Geometry: final body of the model. Coordinates: model frame, mm. A direction names the side the tool comes from. Coordinates: 2 decimals unless noted, no trailing zeros. Write each loop counter-clockwise with the first axis right and the second up, starting at its lowest first coordinate (ties: lowest second). Pieces come first, ordered by that corner, then holes. Notation, with made-up numbers: M 44,-15.5 L 89,-15.5 A25 ccw 89,20.5 Z; hole C 58,30.25 d1. An arc over 180 degrees is marked long. Write item = value, one per line. Start each with the question number.
Item 1: Reachability of faces 1 (the flat face through (0, 0, 10.5)), 2 (the flat face through (32, 0, 7)) from +Z, -Z, +X, -X, +Y, -Y: full face, straight path, thin tool, end or side. Return the list, or none.
Item 2: Pull-direction query (X, two-part tool) for faces 3 (the flat face through (28, 0, 0.5)), 4 (the cylindrical face through (27.45, -19.06, 6.91)), 5 (the cylindrical face through (-30.05, -19.06, 6.91)), 6 (the flat face through (-32, 0, 7)); classes: +X half, -X half, draft (parallel to the pull), parting line (faces both ways), or undercut.
Item 3: Section A-A on z = 3.75. Output: boundary loops of the cut face in (x, y), plus the area to 3 significant figures.
Item 4: Ray query, L1, parallel to X at y = -19, z = 9; L2, parallel to Y at x = 28.75, z = 7.5; L3, parallel to X at y = -15.5, z = 8.75. Return the intervals inside material, ascending. Write a range as [from, to].
Item 5: Section D-D on y = -10. Output: boundary loops of the cut face in (x, z).
Item 6: Section B-B on x = -28.75. Output: boundary loops of the cut face in (y, z), plus the area to 3 significant figures.
Item 7: First-contact query: pin 1 Ø1.5 at (x, z) = (22.5, 4.5) entering from -Y; pin 2 Ø15 at (x, y) = (12.5, -5.5) entering from -Z; pin 3 Ø3.5 at (x, y) = (28.75, -19) entering from +Z. Flat tips, straight axial feed; report the tip coordinate or a pass-through.
Item 8: Section C-C on y = 19. Output: boundary loops of the cut face in (x, z).
from build123d import *

# Parameters (mm, degrees)
SKETCH_W        = 64
SKETCH_H        = 54
PAD_DEPTH       = 3
SKETCH001_W     = 7
SKETCH001_H     = 54
PAD001_DEPTH    = 10
SKETCH002_R     = 1.3
POCKET_DEPTH    = 20
SKETCH003_R     = 1.3
POCKET001_DEPTH = 20


with BuildPart() as part:
    # Sketch → Pad (new body)
    with BuildSketch(Plane.XY):
        Rectangle(SKETCH_W, SKETCH_H)
    extrude(amount=PAD_DEPTH)

    # Sketch001 (on Face5 of Pad) → Pad001 (join)
    with BuildSketch(Plane(origin=(0, 0, 0), x_dir=(1, 0, 0), z_dir=(0, 0, -1))):
        with Locations((28.5, 0)):
            Rectangle(SKETCH001_W, SKETCH001_H)
        with Locations((-28.5, 0)):
            Rectangle(SKETCH001_W, SKETCH001_H)
    extrude(amount=PAD001_DEPTH)

    # Sketch002 (on Face12 of Pad001) → Pocket (cut)
    with BuildSketch(Plane(origin=(0, 0, -10), x_dir=(1, 0, 0), z_dir=(0, 0, -1))):
        with Locations((-28.75, 19)):
            Circle(SKETCH002_R)
        with Locations((-28.75, -19)):
            Circle(SKETCH002_R)
    extrude(amount=-POCKET_DEPTH, mode=Mode.SUBTRACT)

    # Sketch003 (on Face14 of Pocket) → Pocket001 (cut)
    with BuildSketch(Plane(origin=(0, 0, -10), x_dir=(1, 0, 0), z_dir=(0, 0, -1))):
        with Locations((28.75, 19)):
            Circle(SKETCH003_R)
        with Locations((28.75, -19)):
            Circle(SKETCH003_R)
    extrude(amount=-POCKET001_DEPTH, mode=Mode.SUBTRACT)


with BuildPart() as part_1:
    # Body placement: moved
    add(part.part.moved(Location((0, 0, 10.5))))


solid = part_1.part
Responses:
q1.face_1 = -Z, +Y, -Y
q1.face_2 = +Z, -Z, +X, +Y, -Y
q2.face_3 = draft
q2.face_4 = undercut
q2.face_5 = undercut
q2.face_6 = -X half
q3.outline = M -32,-27 L -25,-27 L -25,27 L -32,27 Z; M 25,-27 L 32,-27 L 32,27 L 25,27 Z; hole C -28.75,-19 d2.6; hole C -28.75,19 d2.6; hole C 28.75,-19 d2.6; hole C 28.75,19 d2.6
q3.area = 735 mm²
q4.L1 = [-32, -30.05], [-27.45, -25], [25, 27.45], [30.05, 32]
q4.L2 = [-27, -20.3], [-17.7, 17.7], [20.3, 27]
q4.L3 = [-32, -25], [25, 32]
q5.outline = M -32,0.5 L -25,0.5 L -25,10.5 L 25,10.5 L 25,0.5 L 32,0.5 L 32,13.5 L -32,13.5 Z
q6.outline = M -27,0.5 L -20.3,0.5 L -20.3,13.5 L -27,13.5 Z; M -17.7,0.5 L 17.7,0.5 L 17.7,13.5 L -17.7,13.5 Z; M 20.3,0.5 L 27,0.5 L 27,13.5 L 20.3,13.5 Z
q6.area = 634 mm²
q7.pin_1 = through
q7.pin_2 = 10.5
q7.pin_3 = 13.5
q8.outline = M -32,0.5 L -30.05,0.5 L -30.05,13.5 L -32,13.5 Z; M -27.45,0.5 L -25,0.5 L -25,10.5 L 25,10.5 L 25,0.5 L 27.45,0.5 L 27.45,13.5 L -27.45,13.5 Z; M 30.05,0.5 L 32,0.5 L 32,13.5 L 30.05,13.5 Z
